from build123d import *

# Parameters (mm, degrees)
F1_DEPTH = 25.4
F3_DEPTH = 12.701
F5_DEPTH = 12.701
F7_DEPTH = 50.801


with BuildPart() as f1:
    # F0 (on Front) → F1 (new body)
    with BuildSketch(Plane.XZ):
        Polygon((-31.273121752, 12.7), (-31.273121752, 0), (44.926878248, 0), (44.926878248, 12.7), (19.526878248, 12.7), (19.526878248, 44.45), (-5.873121752, 44.45), (-5.873121752, 12.7), align=None)
    extrude(amount=F1_DEPTH)

    # F2 (on face) → F3 (cut, through all)
    with BuildSketch(Plane.XY.offset(12.7)):
        with BuildLine():
            ThreePointArc((38.576878248, -12.7), (36.7170063085, -8.2098719395), (32.226878248, -6.35))
            Line((32.226878248, -6.35), (32.226878248, -19.05))
            ThreePointArc((32.226878248, -19.05), (36.7170063085, -17.1901280605), (38.576878248, -12.7))
        make_face()
        with BuildLine():
            Line((32.226878248, -19.05), (32.226878248, -6.35))
            ThreePointArc((32.226878248, -6.35), (25.876878248, -12.7), (32.226878248, -19.05))
        make_face()
        with BuildLine():
            Line((44.926878248, 0), (32.226878248, 0))
            ThreePointArc((32.226878248, 0), (41.2071343691, -3.7197438789), (44.926878248, -12.7))
            Line((44.926878248, -12.7), (44.926878248, 0))
        make_face()
        with BuildLine():
            Line((44.926878248, -25.4), (44.926878248, -12.7))
            ThreePointArc((44.926878248, -12.7), (41.2071343691, -21.6802561211), (32.226878248, -25.4))
            Line((32.226878248, -25.4), (44.926878248, -25.4))
        make_face()
    extrude(amount=-F3_DEPTH, mode=Mode.SUBTRACT)

    # F4 (on face) → F5 (cut, through all)
    with BuildSketch(Plane.XY.offset(12.7)):
        with BuildLine():
            ThreePointArc((-12.223121752, -12.7), (-14.0829936915, -8.2098719395), (-18.573121752, -6.35))
            Line((-18.573121752, -6.35), (-18.573121752, -19.05))
            ThreePointArc((-18.573121752, -19.05), (-14.0829936915, -17.1901280605), (-12.223121752, -12.7))
        make_face()
        with BuildLine():
            Line((-18.573121752, -19.05), (-18.573121752, -6.35))
            ThreePointArc((-18.573121752, -6.35), (-24.923121752, -12.7), (-18.573121752, -19.05))
        make_face()
        with BuildLine():
            ThreePointArc((-31.273121752, -12.7), (-27.5533778731, -3.7197438789), (-18.573121752, 0))
            Line((-18.573121752, 0), (-31.273121752, 0))
            Line((-31.273121752, 0), (-31.273121752, -12.7))
        make_face()
        with BuildLine():
            ThreePointArc((-18.573121752, -25.4), (-27.5533778731, -21.6802561211), (-31.273121752, -12.7))
            Line((-31.273121752, -12.7), (-31.273121752, -25.4))
            Line((-31.273121752, -25.4), (-18.573121752, -25.4))
        make_face()
    extrude(amount=-F5_DEPTH, mode=Mode.SUBTRACT)

    # F6 (on face) → F7 (cut, through all)
    with BuildSketch(Plane.YZ.offset(19.526878248)):
        with BuildLine():
            ThreePointArc((-25.4, 31.75), (-21.6802561211, 40.7302561211), (-12.7, 44.45))
            Line((-12.7, 44.45), (-25.4, 44.45))
            Line((-25.4, 44.45), (-25.4, 31.75))
        make_face()
        with BuildLine():
            ThreePointArc((-12.7, 44.45), (-3.7197438789, 40.7302561211), (0, 31.75))
            Line((0, 31.75), (0, 44.45))
            Line((0, 44.45), (-12.7, 44.45))
        make_face()
        with BuildLine():
            Line((-19.05, 31.75), (-6.35, 31.75))
            ThreePointArc((-6.35, 31.75), (-12.7, 38.1), (-19.05, 31.75))
        make_face()
        with BuildLine():
            ThreePointArc((-19.05, 31.75), (-12.7, 25.4), (-6.35, 31.75))
            Line((-6.35, 31.75), (-19.05, 31.75))
        make_face()
    extrude(amount=-F7_DEPTH, mode=Mode.SUBTRACT)


solid = f1.part
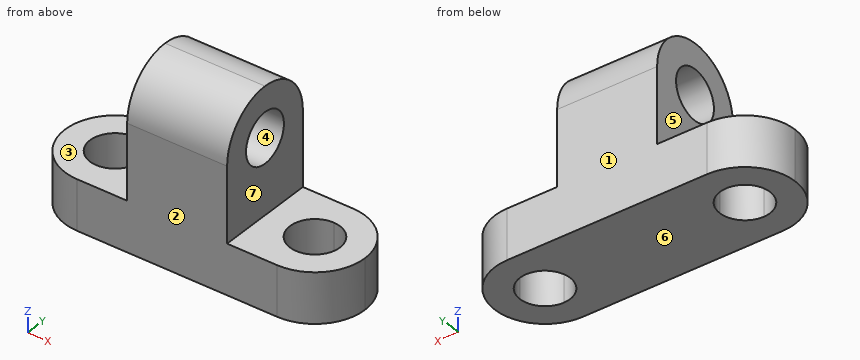
Model file for the job. Use its own axes, mm. Face numbers are marked on the shaded views. A direction names the side the tool comes from. Coordinates: 2 decimals unless noted, no trailing zeros. Write each loop counter-clockwise with the first axis right and the second up, starting at its lowest first coordinate (ties: lowest second). Pieces come first, ordered by that corner, then holes. Notation, with made-up numbers: (7.5, 69.5) - (41.5, 69.5) arc R18 cw to (41.5, 79.5) - close; hole circle Ø2 at (45.5, 1.5). An arc over 180 degrees is marked (long way). Write each question's results on one line, items separated by ' | '. Start each with the question number.
1) Flat gauge pins, fed straight in: P1, Ø1, axis at y = -4, z = 38.5, coming from the -X side; P2, Ø5, axis at y = -7.5, z = 6, coming from the -X side; P3, Ø12.5, axis at x = 32, y = -8.5, coming from the +Z side. Where does each tip first touch, or does it go through?
2) Cut at C-C (y = -9). Write the cut outline in (x, z).
3) Cut at B-B (x = -14). Write the cut outline in (y, z).
4) Probe line 1 along Z through (x, y) = (-0.5, -12.7); line 2 along Y through (x, z) = (0, 31.75); line 3 along X through (y, z) = (-18, 25). List the from-to ranges inside material, lowest first. Write a range as from..to.
5) Mould opens along Y. For the marked faces 1, 2, 3 and 4 say: pulls with the +Y half, pulls with the -Y half, needs draft (parallel to the pull), parting line crosses it, or undercut.
6) 3-axis set-ups, long thin cutter, end or side, ignore diameter. For the marked faces 5, 6 and 7: which of +Z, -Z, +X, -X, +Y, -Y reach the whole face in a straight line?
7) Cut at A-A (z = 33.5). Write the cut outline in (x, y), then the cut area to 3 significant figures.
8) Cut at D-D (x = 9.5). Write the cut outline in (y, z), then the cut area to 3 significant figures.
Returned:
1) P1: x = -5.87 | P2: x = -30.98 | P3: z = 12.7
2) outline: (-30.72, 0) - (-23.73, 0) - (-23.73, 12.7) - (-30.72, 12.7) - close; (-13.41, 0) - (27.07, 0) - (27.07, 12.7) - (19.53, 12.7) - (19.53, 26.59) - (-5.87, 26.59) - (-5.87, 12.7) - (-13.41, 12.7) - close; (-5.87, 36.91) - (19.53, 36.91) - (19.53, 43.9) - (-5.87, 43.9) - close; (37.39, 0) - (44.38, 0) - (44.38, 12.7) - (37.39, 12.7) - close
3) outline: (-25.4, 0) - (-17.11, 0) - (-17.11, 12.7) - (-25.4, 12.7) - close; (-8.29, 0) - (0, 0) - (0, 12.7) - (-8.29, 12.7) - close
4) line 1: 0..25.4, 38.1..44.45 | line 2: -25.4..-19.05, -6.35..0 | line 3: -5.87..19.53
5) face 1: pulls with the +Y half | face 2: pulls with the -Y half | face 3: needs draft | face 4: undercut
6) face 5: +Z, -X, +Y, -Y | face 6: -Z, +X, -X, +Y, -Y | face 7: +Z, +X, +Y, -Y
7) outline: (-5.87, -25.28) - (19.53, -25.28) - (19.53, -18.8) - (-5.87, -18.8) - close; (-5.87, -6.6) - (19.53, -6.6) - (19.53, -0.12) - (-5.87, -0.12) - close | area: 329 mm^2
8) outline: (-25.4, 0) - (0, 0) - (0, 31.75) arc R12.7 ccw to (-25.4, 31.75) - close; hole circle Ø12.7 at (-12.7, 31.75) | area: 933 mm^2
